For this review, take the finished solid that the model builds, in its own axes (mm). A direction names the side the tool comes from. Round coordinates to 2 decimals unless told otherwise and drop trailing zeros. Loops run counter-clockwise (first coordinate to the right, second up) from the corner with the lowest first, then second, coordinate; pieces in that order, holes last. Notation, with made-up numbers: (31, 80) -> (43, 80) arc R11 ccw to (43, 87) -> close; hole circle Ø6 at (8, 35.25). An arc over 180 degrees is marked (long way). Write each question's results on one line, items separated by ' | '.
```python
from build123d import *


with BuildPart() as f1:
    # F0 (on Front) → F1 (revolve)
    with BuildSketch(Plane.XZ):
        Polygon((-9.3218, 35.9664), (-13.2334, 35.9664), (-13.2334, 16.8656), (-28.853873, 16.8656), (-28.853873, 9.0424), (-42.7736, 9.0424), (-42.7736, 0), (0, 0), (0, 16.8656), (-9.3218, 16.8656), align=None)
    revolve(axis=Axis((-21.3868, 0, 0), (1, 0, 0)))

    # F0 (on Front) → F2 (revolve)
    with BuildSketch(Plane.XZ):
        Polygon((-9.3218, 35.9664), (-13.2334, 35.9664), (-13.2334, 16.8656), (-28.853873, 16.8656), (-28.853873, 9.0424), (-42.7736, 9.0424), (-42.7736, 0), (0, 0), (0, 16.8656), (-9.3218, 16.8656), align=None)
    revolve(axis=Axis((0, 0, 0), (-1, 0, 0)))

    # F3: F1 across plane


with BuildPart() as f1_1:
    add(f1.part)
    add(f1.part.mirror(Plane.YZ))


solid = f1_1.part
```
1. Consider section B-B (y = 0). State the section outline as (x, z) points.
Values found:
outline: (-42.77, -9.04) -> (-28.85, -9.04) -> (-28.85, -16.87) -> (-13.23, -16.87) -> (-13.23, -35.97) -> (-9.32, -35.97) -> (-9.32, -16.87) -> (9.32, -16.87) -> (9.32, -35.97) -> (13.23, -35.97) -> (13.23, -16.87) -> (28.85, -16.87) -> (28.85, -9.04) -> (42.77, -9.04) -> (42.77, 9.04) -> (28.85, 9.04) -> (28.85, 16.87) -> (13.23, 16.87) -> (13.23, 35.97) -> (9.32, 35.97) -> (9.32, 16.87) -> (-9.32, 16.87) -> (-9.32, 35.97) -> (-13.23, 35.97) -> (-13.23, 16.87) -> (-28.85, 16.87) -> (-28.85, 9.04) -> (-42.77, 9.04) -> close
2. For pin 1 (6 mm diameter, centred on y = -16.5, z = 19, fed in from -X); pin 2 (6 mm diameter, centred on x = -13, z = -23, fed in from -Y); pin 3 (8 mm diameter, centred on x = 10.5, z = -19.5, fed in from +Y), all flat-tipped, find the tip position at first contact; note any pin that passes through.
Values found:
pin 1: stops at x = -13.23 | pin 2: stops at y = -29.89 | pin 3: stops at y = 32.46
3. Draft analysis for pull direction X (two halves, no side actions). For faces 5 (the face through (-35.911, 8.827, -1.96)), 6 (the face through (9.322, 15.5, -7.5)), 7 (the face through (42.774, 0, 0)), state which applies: released by +X, released by -X, zero draft, split by the parting line, or undercut.
Values found:
face 5: zero draft | face 6: undercut | face 7: released by +X
4. Consider section A-A (z = -28). State the section outline as (x, y) points, plus the area to 3 significant figures.
Values found:
outline: (-13.23, -22.57) -> (-9.32, -22.57) -> (-9.32, 22.57) -> (-13.23, 22.57) -> close; (9.32, -22.57) -> (13.23, -22.57) -> (13.23, 22.57) -> (9.32, 22.57) -> close | area: 353 mm2
5. Tool access review of faces 1 (the face through (-42.774, 0, 0)), 2 (the face through (-9.322, 15.5, -7.5)), 3 (the face through (28.854, 7, 7)), 4 (the face through (-21.15, -16.72, -2.2)): name each direction out of +Z, -Z, +X, -X, +Y, -Y from which nothing blocks a thin tool from reaching the whole face with its end or side.
Values found:
face 1: +Z, -Z, -X, +Y, -Y | face 2: none | face 3: +X | face 4: -X
6. To check wall thickness, follow probe 1 along X at (y, z) = (15.5, -20); probe 2 along X at (y, z) = (-9.5, 8.5); probe 3 along Z at (x, y) = (-27.5, 7.5). State the ranges of each line that lie inside material, in increasing order.
Values found:
probe 1: x = -13.23 to -9.32, 9.32 to 13.23 | probe 2: x = -28.85 to 28.85 | probe 3: z = -15.11 to 15.11
7. Consider section C-C (x = -31.5). State the section outline as (y, z) points.
Values found:
outline: circle Ø18.08 at (0, 0)
8. Consider section D-D (y = -29). State the section outline as (x, z) points, plus the area to 3 significant figures.
Values found:
outline: (-13.23, -21.27) -> (-9.32, -21.27) -> (-9.32, 21.27) -> (-13.23, 21.27) -> close; (9.32, -21.27) -> (13.23, -21.27) -> (13.23, 21.27) -> (9.32, 21.27) -> close | area: 333 mm2
